from build123d import *

# Parameters (mm, degrees)
SKETCH2_R                     = 11.25
BOSS_EXTRUDE1_DEPTH           = 9
BOSS_EXTRUDE2_DEPTH           = 2
CSK_FOR_M5_SFHCS1_D           = 5.3
CSK_FOR_M5_SFHCS1_CSINK_D     = 11.2
CSK_FOR_M5_SFHCS1_CSINK_ANGLE = 90
FILLET1_R                     = 4
FILLET2_R                     = 1.5


with BuildPart() as part:
    # Sketch2 → Boss-Extrude1 (new body)
    with BuildSketch(Plane(origin=(0, 0, 0), x_dir=(1, 0, 0), z_dir=(0, 1, 0))):
        with BuildLine():
            Line((-15, 0), (-15, 31))
            Line((-15, 31), (15, 31))
            Line((15, 31), (15, 0))
            ThreePointArc((15, 0), (0, -15), (-15, 0))
        make_face()
        with Locations(Location((0, 0, 0), (0, 0, 270))):
            Circle(SKETCH2_R, mode=Mode.SUBTRACT)
    extrude(amount=BOSS_EXTRUDE1_DEPTH)

    # Sketch2_3 → Boss-Extrude2 (add)
    with BuildSketch(Plane(origin=(0, 0, 0), x_dir=(1, 0, 0), z_dir=(0, 1, 0))):
        with BuildLine():
            ThreePointArc((-9, 0), (0, 9), (9, 0))
            Line((9, 0), (11.25, 0))
            ThreePointArc((11.25, 0), (0, 11.25), (-11.25, 0))
            Line((-11.25, 0), (-9, 0))
        make_face()
        with BuildLine():
            Line((11.25, 0), (9, 0))
            ThreePointArc((9, 0), (0, -9), (-9, 0))
            Line((-9, 0), (-11.25, 0))
            ThreePointArc((-11.25, 0), (0, -11.25), (11.25, 0))
        make_face()
    extrude(amount=BOSS_EXTRUDE2_DEPTH)

    # CSK for M5 SFHCS1 (through all)
    with Locations(Plane(origin=(7.4, 0, -21), x_dir=(0, 0, -1), z_dir=(0, -1, 0))):
        with Locations((0, 0), (0, -14.9)):
            CounterSinkHole(CSK_FOR_M5_SFHCS1_D / 2, CSK_FOR_M5_SFHCS1_CSINK_D / 2, counter_sink_angle=CSK_FOR_M5_SFHCS1_CSINK_ANGLE)

    # Fillet1
    fillet1_edges = [part.edges().sort_by_distance(p)[0] for p in [
        (-15, 4.5, -31),
        (15, 4.5, -31),
    ]]
    fillet(fillet1_edges, radius=FILLET1_R)

    # Fillet2
    fillet2_edges = [part.edges().sort_by_distance(p)[0] for p in [
        (15, 9, -13.5),
        (9, 2, 0),
        (-15, 9, -13.5),
        (0, 9, -11.25),
        (0, 0, -31),
        (13.828427125, 0, -29.828427125),
        (-13.828427125, 0, -29.828427125),
        (0, 9, -31),
        (13.828427125, 9, -29.828427125),
        (-13.828427125, 9, -29.828427125),
        (0, 9, 15),
        (-15, 0, -13.5),
        (15, 0, -13.5),
        (0, 0, 15),
    ]]
    fillet(fillet2_edges, radius=FILLET2_R)


solid = part.part
Check sheet for the modelled part. Datum: model origin and axes. Units: mm. A direction names the side the tool comes from. Give positions to 0.01 mm unless a question says otherwise; leave off trailing zeros. Write each loop counter-clockwise with the first axis right and the second up, starting at its lowest first coordinate (ties: lowest second). Pieces come first, ordered by that corner, then holes. Notation, with made-up numbers: (-18.5, 71.25) -> (5.5, 71.25) arc R23 cw to (5.5, 98.25) -> close; hole circle Ø5 at (-10, 66.25). An arc over 180 degrees is marked (long way). Write item = value, one per line.
Item 1: Sectioned sample at B-B on y = 6.75. Record the boundary of the cut face in (x, z), and give its area (3 significant figures).
Output:
outline = (-15, -27) arc R4 ccw to (-11, -31) -> (11, -31) arc R4 ccw to (15, -27) -> (15, 0) arc R15 ccw to (-15, 0) -> close; hole circle Ø22.5 at (0, 0); hole circle Ø5.3 at (-7.5, -21); hole circle Ø5.3 at (7.4, -21)
area = 835 mm^2
Item 2: Tool access check on faces 4 (the cylindrical face through (3.38, 4.71, 10.73)), 5 (the cylindrical face through (14.55, 8.57, -13.31)). Record the directions out of +Z, -Z, +X, -X, +Y, -Y that give a thin tool (end or side, any length) a straight path to the whole face; none if there is none.
Output:
face_4 = +Y
face_5 = +Z, -Z, +X, +Y
Item 3: Release check for a two-part mould opening along Z. For faces 1 (the cylindrical face through (-1.172, 0.246, 8.923)), 2 (the cylindrical face through (0.15, 0.45, -30.57)), 3 (the cylindrical face through (-14.55, 8.57, -13.69)) record: +Z half, -Z half, draft (parallel to the pull), parting line (faces both ways), or undercut.
Output:
face_1 = undercut
face_2 = -Z half
face_3 = draft
Item 4: Sectioned sample at C-C on x = -7.5. Count the separate pieces of the cut face and the enclosed holes in it, and give its area (3 significant figures).
Output:
separate_pieces = 3
enclosed_holes = 0
area = 197 mm^2
Item 5: Gauge pin test, flat ends, axial feed: pin 1 (4 mm diameter, centred on x = -6, z = -5, fed in from +Y); pin 2 (11 mm diameter, centred on x = -3, z = 0.5, fed in from +Y); pin 3 (10 mm diameter, centred on x = -10.5, z = 8, fed in from -Y); pin 4 (4 mm diameter, centred on y = 6.5, z = 3, fed in from +X). Record the tip position at first contact, or that the pin passes through.
Output:
pin_1 = 1.83
pin_2 = through
pin_3 = 0
pin_4 = 14.97
Item 6: Scan lines: probe 1 along X at (y, z) = (6.25, -21); probe 2 along Z at (x, y) = (-7.5, 4.5); probe 3 along Z at (x, y) = (-6.5, 7.5). Record each from-to range of solid material in increasing order. Write a range as from..to.
Output:
probe_1 = -15..-10.15, -4.85..4.75, 10.05..15
probe_2 = -31..-23.65, -18.35..-8.39, 8.39..12.99
probe_3 = -31..-23.45, -18.55..-9.18, 9.18..13.52
Item 7: Sectioned sample at A-A on x = 0. Record the boundary of the cut face in (y, z).
Output:
outline = (0, -29.5) arc R1.5 ccw to (1.5, -31) -> (7.5, -31) arc R1.5 ccw to (9, -29.5) -> (9, -12.75) arc R1.5 ccw to (7.5, -11.25) -> (2, -11.25) -> (2, -10.5) arc R1.5 ccw to (0.5, -9) -> (0, -9) -> close; (0, 9) -> (0.5, 9) arc R1.5 ccw to (2, 10.5) -> (2, 11.25) -> (7.5, 11.25) arc R1.5 ccw to (9, 12.75) -> (9, 13.5) arc R1.5 ccw to (7.5, 15) -> (1.5, 15) arc R1.5 ccw to (0, 13.5) -> close
